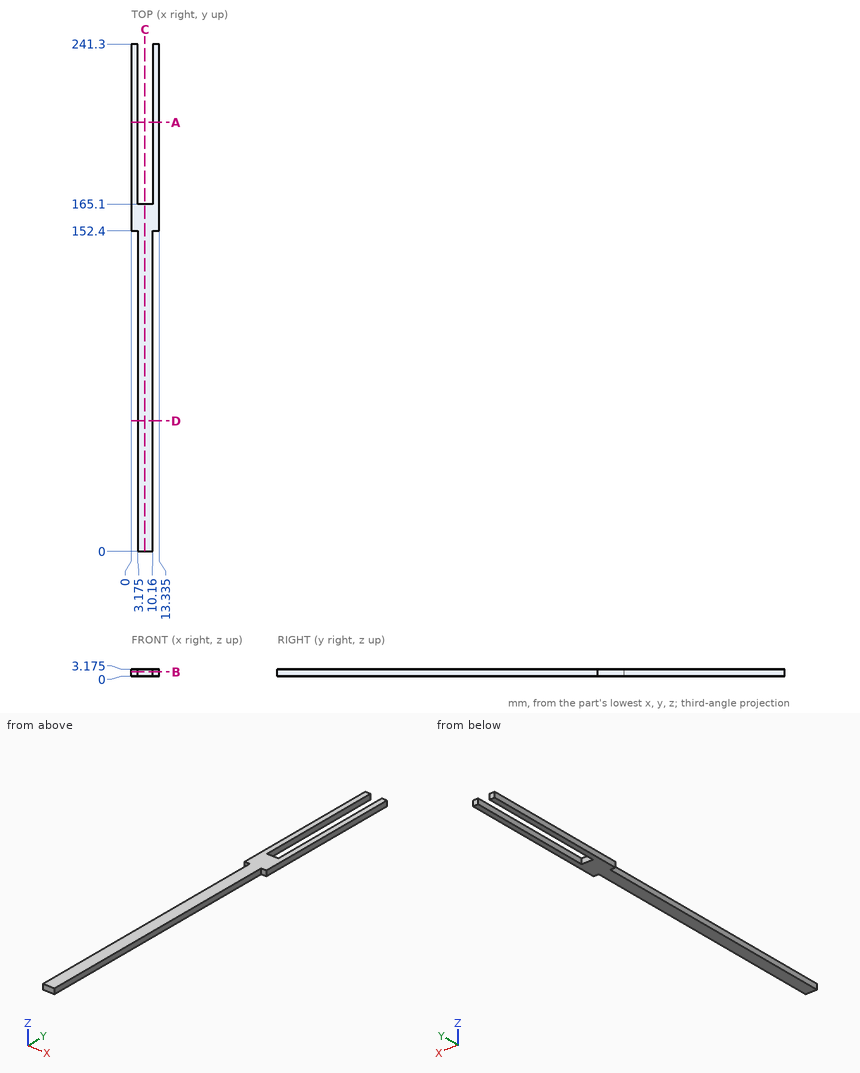
Here's the drawing with two shaded views (mm, measured from the low corner). I have some questions. Coordinates: 2 decimals unless noted, no trailing zeros. Order: outer loops, then holes, each group sorted by start corner. A loop starts at its lowest first (then second) coordinate and runs counter-clockwise, first axis right, second up.
Item 1: If we section it at B-B on z = 2: List the corners of the cut face in (x, y) for me (3 decimals).
Result sheet:
outline: (0, 152.4) - (3.175, 152.4) - (3.175, 0) - (10.16, 0) - (10.16, 152.4) - (13.335, 152.4) - (13.335, 241.3) - (10.16, 241.3) - (10.16, 165.1) - (3.175, 165.1) - (3.175, 241.3) - (0, 241.3) - close
Item 2: For P1, Ø1, axis at x = 8, z = 2, coming from the +Y side; P2, Ø1, axis at y = 54.5, z = 1.5, coming from the -X side (3 decimals), each with a flat end and sliding along its axis, tell me the tip position at first contact or that it passes through.
Result sheet:
P1: stops at y = 165.1
P2: stops at x = 3.175
Item 3: I need wall thicknesses on line 1 (X direction, y = 211.5, z = 2.7) (3 decimals); line 2 (Y direction, x = 9.25, z = 1.45); line 3 (X direction, y = 61, z = 0.35) (3 decimals). Which ranges of each line are inside material? Lowest first, please.
Result sheet:
line 1: x = 0 to 3.175, 10.16 to 13.335
line 2: y = 0 to 165.1
line 3: x = 3.175 to 10.16
Item 4: If we section it at A-A on y = 204: List the corners of the cut face in (x, z) for me (3 decimals), plus the area to 3 significant figures.
Result sheet:
outline: (0, 0) - (3.175, 0) - (3.175, 3.175) - (0, 3.175) - close; (10.16, 0) - (13.335, 0) - (13.335, 3.175) - (10.16, 3.175) - close
area: 20.2 mm2
Item 5: If we section it at C-C on x = 6.5: List the corners of the cut face in (y, z) for me (3 decimals).
Result sheet:
outline: (0, 0) - (165.1, 0) - (165.1, 3.175) - (0, 3.175) - close
Item 6: If we section it at D-D on y = 62: List the corners of the cut face in (x, z) for me (3 decimals), plus the area to 3 significant figures.
Result sheet:
outline: (3.175, 0) - (10.16, 0) - (10.16, 3.175) - (3.175, 3.175) - close
area: 22.2 mm2
